from build123d import *

# Parameters (mm, degrees)
SKETCH1_R            = 55
SKETCH1_R_2          = 4
BOSS_EXTRUDE1_DEPTH  = 10
CUT_SWEEP1_PROFILE_R = 2


with BuildPart() as part:
    # Sketch1 → Boss-Extrude1 (new body)
    with BuildSketch(Plane.XY):
        with BuildLine():
            ThreePointArc((-42.468063511, -112.979478614), (-39.624142049, -114.008010127), (-36.755344443, -114.964967103))
            ThreePointArc((-36.755344443, -114.964967103), (0, -90.746115822), (36.755344443, -114.964967103))
            ThreePointArc((36.755344443, -114.964967103), (39.624142049, -114.008010127), (42.468063511, -112.979478614))
            Line((42.468063511, -112.979478614), (27.935607979, -77.895027374))
            ThreePointArc((27.935607979, -77.895027374), (30.100392379, -72.668775514), (35.326644239, -74.833559915))
            Line((35.326644239, -74.833559915), (49.859099771, -109.918011155))
            ThreePointArc((49.859099771, -109.918011155), (52.597337529, -108.634336612), (55.302554537, -107.282461138))
            ThreePointArc((55.302554537, -107.282461138), (64.167193864, -64.167193864), (107.282461138, -55.302554537))
            ThreePointArc((107.282461138, -55.302554537), (108.634336612, -52.597337529), (109.918011155, -49.859099771))
            Line((109.918011155, -49.859099771), (74.833559915, -35.326644239))
            ThreePointArc((74.833559915, -35.326644239), (72.668775514, -30.100392379), (77.895027374, -27.935607979))
            Line((77.895027374, -27.935607979), (112.979478614, -42.468063511))
            ThreePointArc((112.979478614, -42.468063511), (114.008010127, -39.624142049), (114.964967103, -36.755344443))
            ThreePointArc((114.964967103, -36.755344443), (90.746115822, 0), (114.964967103, 36.755344443))
            ThreePointArc((114.964967103, 36.755344443), (114.008010127, 39.624142049), (112.979478614, 42.468063511))
            Line((112.979478614, 42.468063511), (77.895027374, 27.935607979))
            ThreePointArc((77.895027374, 27.935607979), (72.668775514, 30.100392379), (74.833559915, 35.326644239))
            Line((74.833559915, 35.326644239), (109.918011155, 49.859099771))
            ThreePointArc((109.918011155, 49.859099771), (108.634336612, 52.597337529), (107.282461138, 55.302554537))
            ThreePointArc((107.282461138, 55.302554537), (64.167193864, 64.167193864), (55.302554537, 107.282461138))
            ThreePointArc((55.302554537, 107.282461138), (52.597337529, 108.634336612), (49.859099771, 109.918011155))
            Line((49.859099771, 109.918011155), (35.326644239, 74.833559915))
            ThreePointArc((35.326644239, 74.833559915), (30.100392379, 72.668775514), (27.935607979, 77.895027374))
            Line((27.935607979, 77.895027374), (42.468063511, 112.979478614))
            ThreePointArc((42.468063511, 112.979478614), (39.624142049, 114.008010127), (36.755344443, 114.964967103))
            ThreePointArc((36.755344443, 114.964967103), (0, 90.746115822), (-36.755344443, 114.964967103))
            ThreePointArc((-36.755344443, 114.964967103), (-39.624142049, 114.008010127), (-42.468063511, 112.979478614))
            Line((-42.468063511, 112.979478614), (-27.935607979, 77.895027374))
            ThreePointArc((-27.935607979, 77.895027374), (-30.100392379, 72.668775514), (-35.326644239, 74.833559915))
            Line((-35.326644239, 74.833559915), (-49.859099771, 109.918011155))
            ThreePointArc((-49.859099771, 109.918011155), (-52.597337529, 108.634336612), (-55.302554537, 107.282461138))
            ThreePointArc((-55.302554537, 107.282461138), (-64.167193864, 64.167193864), (-107.282461138, 55.302554537))
            ThreePointArc((-107.282461138, 55.302554537), (-108.634336612, 52.597337529), (-109.918011155, 49.859099771))
            Line((-109.918011155, 49.859099771), (-74.833559915, 35.326644239))
            ThreePointArc((-74.833559915, 35.326644239), (-72.668775514, 30.100392379), (-77.895027374, 27.935607979))
            Line((-77.895027374, 27.935607979), (-112.979478614, 42.468063511))
            ThreePointArc((-112.979478614, 42.468063511), (-114.008010127, 39.624142049), (-114.964967103, 36.755344443))
            ThreePointArc((-114.964967103, 36.755344443), (-90.746115822, 0), (-114.964967103, -36.755344443))
            ThreePointArc((-114.964967103, -36.755344443), (-114.008010127, -39.624142049), (-112.979478614, -42.468063511))
            Line((-112.979478614, -42.468063511), (-77.895027374, -27.935607979))
            ThreePointArc((-77.895027374, -27.935607979), (-72.668775514, -30.100392379), (-74.833559915, -35.326644239))
            Line((-74.833559915, -35.326644239), (-109.918011155, -49.859099771))
            ThreePointArc((-109.918011155, -49.859099771), (-108.634336612, -52.597337529), (-107.282461138, -55.302554537))
            ThreePointArc((-107.282461138, -55.302554537), (-64.167193864, -64.167193864), (-55.302554537, -107.282461138))
            ThreePointArc((-55.302554537, -107.282461138), (-52.597337529, -108.634336612), (-49.859099771, -109.918011155))
            Line((-49.859099771, -109.918011155), (-35.326644239, -74.833559915))
            ThreePointArc((-35.326644239, -74.833559915), (-30.100392379, -72.668775514), (-27.935607979, -77.895027374))
            Line((-27.935607979, -77.895027374), (-42.468063511, -112.979478614))
        make_face()
        Circle(SKETCH1_R, mode=Mode.SUBTRACT)
        with Locations((-78, -0.18)):
            Circle(SKETCH1_R_2, mode=Mode.SUBTRACT)
        with Locations((0, -78)):
            Circle(SKETCH1_R_2, mode=Mode.SUBTRACT)
        with Locations((77.82, 0)):
            Circle(SKETCH1_R_2, mode=Mode.SUBTRACT)
        with Locations((-0.18, 77.82)):
            Circle(SKETCH1_R_2, mode=Mode.SUBTRACT)
    extrude(amount=BOSS_EXTRUDE1_DEPTH)

    # Cut-Sweep1: sweep along a path in Sketch6
    with BuildLine(Plane(origin=(0, 0, 10), x_dir=(-1, 0, 0), z_dir=(0, 0, -1))) as cut_sweep1_path:
        CenterArc((0, 0), 65, 0, 360)
    # Cut-Sweep1 profile (on start of the path) → Cut-Sweep1 (sweep, cut)
    with BuildSketch(Plane(origin=(-65, 0, 10), x_dir=(0, 0, 1), z_dir=(0, 1, 0))):
        Circle(CUT_SWEEP1_PROFILE_R)
    sweep(path=cut_sweep1_path.line, mode=Mode.SUBTRACT)


solid = part.part
Input: part model. Units: mm. Frame: model coordinates. A direction names the side the tool comes from. Coordinates: 2 decimals unless noted, no trailing zeros. Order: outer loops, then holes, each group sorted by start corner. A loop starts at its lowest first (then second) coordinate and runs counter-clockwise, first axis right, second up. Notation, with made-up numbers: M 16,45.5 L 63,45.5 A25 cw 63,73.5 Z; hole C 74,3.5 d6. An arc over 180 degrees is marked long. Write item = value, one per line. Start each with the question number.
(1) Reachability of faces 1 (the cylindrical face through (-39.584, 114.022, 4.93)), 2 (the flat face through (-35.304, 95.683, 4.93)) from +Z, -Z, +X, -X, +Y, -Y: full face, straight path, thin tool, end or side. Return the list, or none.
(2) First-contact query: P1, Ø4, axis at y = 4, z = 8, coming from the -X side; P2, Ø3, axis at x = 7.5, z = 1, coming from the +Y side; P3, Ø5, axis at x = -66, y = 8, coming from the +Z side; P4, Ø1, axis at x = -41, z = 3.5, coming from the -Y side. Flat tips, straight axial feed; report the tip coordinate or a pass-through.
(3) Pull-direction query (Y, two-part tool) for faces 3 (the cylindrical face through (90.75, -0.65, 4.93)), 4 (the cylindrical face through (52.559, -108.653, 4.93)), 5 (the cylindrical face through (0.65, 90.75, 4.93)); classes: released by +Y, released by -Y, zero draft, split by the parting line, or undercut.
(4) Section B-B on z = 1.5. Give the number of separate pieces and of enclosed holes in the cut face, and give its area (3 significant figures).
(5) Section A-A on x = 0. Output: boundary loops of the cut face in (y, z).
(6) Line query: line 1 along Y through (x, z) = (-0.5, 3.5); line 2 along Y through (x, z) = (77.82, 4); line 3 along X through (y, z) = (-88, 3.5). Output: solid intervals per line, ascending. Write a range as [from, to].
Result set:
q1.face_1 = +Z, -Z, -X, +Y
q1.face_2 = +Z, -Z
q2.P1 = -91.2
q2.P2 = 91.77
q2.P3 = 10
q2.P4 = -113.7
q3.face_3 = undercut
q3.face_4 = released by -Y
q3.face_5 = released by +Y
q4.separate_pieces = 1
q4.enclosed_holes = 5
q4.area = 20,900 mm²
q5.outline = M -90.75,0 L -82,0 L -82,10 L -90.75,10 Z; M -74,0 L -55,0 L -55,10 L -63,10 A2 cw -67,10 L -74,10 Z; M 55,0 L 73.82,0 L 73.82,10 L 67,10 A2 cw 63,10 L 55,10 Z; M 81.82,0 L 90.75,0 L 90.75,10 L 81.82,10 Z
q6.line_1 = [-90.75, -81.97], [-74.03, -55], [55, 73.83], [81.81, 90.75]
q6.line_2 = [-55.22, -36.56], [-27.91, -4], [4, 27.91], [36.56, 55.22]
q6.line_3 = [-52.7, -40.78], [-32.12, 32.12], [40.78, 52.7]
